The listing builds one solid part. Answer for the finished solid, in the listing's coordinates (mm). Face numbers are marked on the shaded views. A direction names the side the tool comes from. Round coordinates to 2 decimals unless told otherwise and drop trailing zeros. Write each loop counter-clockwise with the first axis right and the second up, starting at its lowest first coordinate (ties: lowest second). Pieces come first, ordered by that corner, then holes.
Item 1: Find section C-C on x = -14. Give the vertices of the cut face in (y, z), then the cut area to 3 significant figures.
Item 2: Find section D-D on z = 38.5. Give the vertices of the cut face in (x, y), then the cut area to 3 significant figures.
Item 3: Each of these flat-tipped pins is pushed along its axis until it touches: pin 1 (2 mm diameter, centred on x = -21, y = -2.5, fed in from +Z); pin 2 (1.5 mm diameter, centred on x = -38.5, y = -10, fed in from -Z); pin 3 (5 mm diameter, centred on y = -6, z = 37, fed in from -X); pin 4 (18.5 mm diameter, centred on x = -23.75, z = 51.83, fed in from -Y). Where does it stop, or does it pass through?
Item 4: Find section B-B on x = -23.75. Give the vertices of the cut face in (y, z).
Item 5: Find the intervals of material crossed by probe 1 along X at (y, z) = (-6, 9); probe 2 along Z at (x, y) = (-23.75, -12.75); probe 3 along X at (y, z) = (-5.75, 34), in increasing order.
Item 6: For a pull along X with two mould halves and no side action, classify the marked faces 1, 2, 3 and 4 as +X half, -X half, draft (parallel to the pull), parting line (faces both ways), or undercut.
Item 7: Find section A-A on y = -8.5. Give the vertices of the cut face in (x, z).
Item 8: A tool of negligible diameter and unlimited length cuts with its end or side. For the marked faces 5, 6 and 7, from which of +Z, -Z, +X, -X, +Y, -Y can it reach the whole face along a straight path? Write none if from no direction.
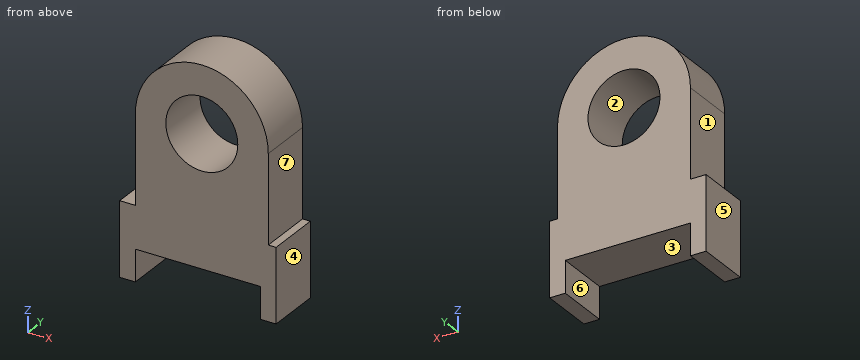
```python
from build123d import *

# Parameters (mm, degrees)
F0_R     = 11.509602
F1_DEPTH = 17.5


with BuildPart() as f1:
    # F0 (on Front) → F1 (new body)
    with BuildSketch(Plane.XZ):
        with BuildLine():
            Line((-5, 0), (0, 0))
            Line((0, 0), (0, 23.633176))
            Line((0, 23.633176), (-2.5, 23.633176))
            Line((-2.5, 23.633176), (-2.5, 51.83411))
            ThreePointArc((-2.5, 51.83411), (-23.75, 73.08411), (-45, 51.83411))
            Line((-45, 51.83411), (-45, 23.633176))
            Line((-45, 23.633176), (-50, 23.633176))
            Line((-50, 23.633176), (-50, 0))
            Line((-50, 0), (-45, 0))
            Line((-45, 0), (-45, 10.128504))
            Line((-45, 10.128504), (-5, 10.128504))
            Line((-5, 10.128504), (-5, 0))
        make_face()
        with Locations((-23.75, 51.83411)):
            Circle(F0_R, mode=Mode.SUBTRACT)
    extrude(amount=F1_DEPTH)


solid = f1.part
```
Check values:
1. outline: (-17.5, 10.13) - (0, 10.13) - (0, 45.72) - (-17.5, 45.72) - close; (-17.5, 57.95) - (0, 57.95) - (0, 70.72) - (-17.5, 70.72) - close
1. area: 846 mm2
2. outline: (-45, -17.5) - (-2.5, -17.5) - (-2.5, 0) - (-45, 0) - close
2. area: 744 mm2
3. pin 1: stops at z = 73.01
3. pin 2: stops at z = 10.13
3. pin 3: stops at x = -45
3. pin 4: passes through
4. outline: (-17.5, 10.13) - (0, 10.13) - (0, 40.32) - (-17.5, 40.32) - close; (-17.5, 63.34) - (0, 63.34) - (0, 73.08) - (-17.5, 73.08) - close
5. probe 1: x = -50 to -45, -5 to 0
5. probe 2: z = 10.13 to 40.32, 63.34 to 73.08
5. probe 3: x = -45 to -2.5
6. face 1: -X half
6. face 2: undercut
6. face 3: undercut
6. face 4: +X half
7. outline: (-50, 0) - (-45, 0) - (-45, 10.13) - (-5, 10.13) - (-5, 0) - (0, 0) - (0, 23.63) - (-2.5, 23.63) - (-2.5, 51.83) arc R21.25 ccw to (-45, 51.83) - (-45, 23.63) - (-50, 23.63) - close; hole circle Ø23.02 at (-23.75, 51.83)
8. face 5: +Z, -Z, -X, +Y, -Y
8. face 6: -Z, +Y, -Y
8. face 7: +Z, +X, +Y, -Y
